```python
from build123d import *

# Parameters (mm, degrees)
F0_R     = 37.5
F1_DEPTH = 23
F2_R     = 34.5
F2_R_2   = 6
F3_DEPTH = 10
F4_R     = 34.5
F4_R_2   = 6
F5_DEPTH = 10


with BuildPart() as f1:
    # F0 (on Top) → F1 (new body)
    with BuildSketch(Plane.XY):
        Circle(F0_R)
    extrude(amount=F1_DEPTH)

    # F2 (on face) → F3 (cut)
    with BuildSketch(Plane.XY.offset(23)):
        Circle(F2_R)
        Circle(F2_R_2, mode=Mode.SUBTRACT)
    extrude(amount=-F3_DEPTH, mode=Mode.SUBTRACT)

    # F4 (on face) → F5 (cut)
    with BuildSketch(Plane(origin=(0, 0, 0), x_dir=(1, 0, 0), z_dir=(0, 0, -1))):
        Circle(F4_R)
        Circle(F4_R_2, mode=Mode.SUBTRACT)
    extrude(amount=-F5_DEPTH, mode=Mode.SUBTRACT)


solid = f1.part
```
Can you work these out from the model? Positions are in its coordinate system, mm. A direction names the side the tool comes from. Round coordinates to 2 decimals unless told otherwise and drop trailing zeros. Order: outer loops, then holes, each group sorted by start corner. A loop starts at its lowest first (then second) coordinate and runs counter-clockwise, first axis right, second up. Notation, with made-up numbers: (-29.5, -5.5) -> (29.5, -5.5) arc R16 cw to (29.5, 13.5) -> close; hole circle Ø3 at (-14.75, 35.5). An arc over 180 degrees is marked (long way). Return JSON: item names as keys, results as strings. Group by question number.
1. Will these pins go through, and if not, where does the flat tip stop? pin 1 (1 mm diameter, centred on y = -24.5, z = 9.5, fed in from +X); pin 2 (1 mm diameter, centred on x = -6.5, z = 17, fed in from +Y); pin 3 (3 mm diameter, centred on x = -22.5, z = 7, fed in from -Y).
2. If we section it at D-D, the plane x = -25: Write out the boundary of the cut face in (y, z), then the cut area to 3 significant figures.
3. If we section it at B-B, the plane x = 0: Write out the boundary of the cut face in (y, z), then the cut area to 3 significant figures.
4. If we section it at A-A, the plane z = 5: Write out the boundary of the cut face in (x, y), then the cut area to 3 significant figures.
5. Which directions (+Z, -Z, +X, -X, +Y, -Y) give clear straight access to the entire face, cutting with the end or side of a thin tool? Please do faces 5 (the face through (0, -7, 13)), 6 (the face through (32.907, -10.363, 4.93)), 7 (the face through (11, -33, 23)).
6. We'd pull the mould along X, two halves only. Please class faces 1 (the face through (-6, 0, 18)), 2 (the face through (0, 0, 23)), 3 (the face through (-6, 0, 5)), 4 (the face through (-4.88, 37.18, 11.34)): released by +X, released by -X, zero draft, split by the parting line, or undercut.
7. I need wall thicknesses on line 1 (Y direction, x = 0, z = 16.75); line 2 (Z direction, x = 12, y = 4.5); line 3 (X direction, y = 24, z = 4.25). Which ranges of each line are inside material? Lowest first, please. Write a range as [from, to].
Output values:
{
 "1": {"pin 1": "x = 28.81", "pin 2": "y = 37.02", "pin 3": "y = -31.07"},
 "2": {"outline": "(-27.95, 0) -> (-23.77, 0) -> (-23.77, 10) -> (23.77, 10) -> (23.77, 0) -> (27.95, 0) -> (27.95, 23) -> (23.77, 23) -> (23.77, 13) -> (-23.77, 13) -> (-23.77, 23) -> (-27.95, 23) -> close", "area": "335 mm²"},
 "3": {"outline": "(-37.5, 0) -> (-34.5, 0) -> (-34.5, 10) -> (-6, 10) -> (-6, 0) -> (6, 0) -> (6, 10) -> (34.5, 10) -> (34.5, 0) -> (37.5, 0) -> (37.5, 23) -> (34.5, 23) -> (34.5, 13) -> (6, 13) -> (6, 23) -> (-6, 23) -> (-6, 13) -> (-34.5, 13) -> (-34.5, 23) -> (-37.5, 23) -> close", "area": "585 mm²"},
 "4": {"outline": "circle Ø75 at (0, 0); circle Ø12 at (0, 0); hole circle Ø69 at (0, 0)", "area": "792 mm²"},
 "5": {"face 5": "+Z", "face 6": "-Z", "face 7": "+Z, +X, -X, +Y, -Y"},
 "6": {"face 1": "undercut", "face 2": "zero draft", "face 3": "undercut", "face 4": "split by the parting line"},
 "7": {"line 1": "[-37.5, -34.5], [-6, 6], [34.5, 37.5]", "line 2": "[10, 13]", "line 3": "[-28.81, -24.78], [24.78, 28.81]"}
}
